```python
from build123d import *

# Parameters (mm, degrees)
F0_R     = 9.3155
F1_DEPTH = 11
F2_R     = 10.4775
F3_DEPTH = 19
F4_R     = 9.3155
F5_DEPTH = 11


with BuildPart() as f1:
    # F0 (on Front) → F1 (new body)
    with BuildSketch(Plane.XZ):
        Polygon((13.5, -5.591883), (13.5, 5.591883), (5.591883, 13.5), (-5.591883, 13.5), (-13.5, 5.591883), (-13.5, -5.591883), (-5.591883, -13.5), (5.591883, -13.5), align=None)
        Circle(F0_R, mode=Mode.SUBTRACT)
    extrude(amount=F1_DEPTH)

    # F2 (on face) → F3 (join)
    with BuildSketch(Plane(origin=(0, 0, 0), x_dir=(-1, 0, 0), z_dir=(0, 1, 0))):
        Polygon((21, -8.698485), (21, 8.698485), (8.698485, 21), (-8.698485, 21), (-21, 8.698485), (-21, -8.698485), (-8.698485, -21), (8.698485, -21), align=None)
        Circle(F2_R, mode=Mode.SUBTRACT)
    extrude(amount=F3_DEPTH)

    # F4 (on face) → F5 (join)
    with BuildSketch(Plane(origin=(0, 19, 0), x_dir=(-1, 0, 0), z_dir=(0, 1, 0))):
        Polygon((13.5, -5.591883), (13.5, 5.591883), (5.591883, 13.5), (-5.591883, 13.5), (-13.5, 5.591883), (-13.5, -5.591883), (-5.591883, -13.5), (5.591883, -13.5), align=None)
        Circle(F4_R, mode=Mode.SUBTRACT)
    extrude(amount=F5_DEPTH)


solid = f1.part
```
Work out the finished part from the listing and answer in its coordinate system (mm). A direction names the side the tool comes from. Give positions to 0.01 mm unless a question says otherwise; leave off trailing zeros. Order: outer loops, then holes, each group sorted by start corner. A loop starts at its lowest first (then second) coordinate and runs counter-clockwise, first axis right, second up. Notation, with made-up numbers: (66.5, -9.5) - (100.5, -9.5) arc R11 cw to (100.5, -3.5) - close; hole circle Ø8 at (24.25, 49). An arc over 180 degrees is marked (long way). One line per item, written item: value. Start each with the question number.
1. Section A-A, the plane x = 0 is taken. Write down the section's boundary in (y, z).
2. Section C-C, the plane y = -4 is taken. Write down the section's boundary in (x, z), then the cut area to 3 significant figures.
3. Consider line 1 (Z direction, x = 0, y = -5.5); line 2 (Z direction, x = 0, y = 10.5); line 3 (X direction, y = 24.5, z = 1). Determine where each line is inside the solid, lowest interval first.
4. Each of these flat-tipped pins is pushed along its axis until it touches: pin 1 Ø10 at (y, z) = (25, 8) entering from -X; pin 2 Ø3 at (x, y) = (0, -6) entering from -Z; pin 3 Ø3 at (x, y) = (13.5, 11) entering from +Z; pin 4 Ø6.5 at (x, z) = (0, 3) entering from +Y. Where does it stop, or does it pass through?
5. Which of the six approach directions +Z, -Z, +X, -X, +Y, -Y give full straight-line access (tool end or side, diameter ignored) to faces 4 (the face through (9.49, 24.42, 9.6)), 5 (the face through (-9.49, -5.42, 9.6)), 6 (the face through (0, -5, -13.5))?
6. Section B-B, the plane z = 0 is taken. Write down the section's boundary in (x, y), then the cut area to 3 significant figures.
7. Section D-D, the plane y = 17 is taken. Write down the section's boundary in (x, z) (1 decimal), then the cut area to 3 significant figures.
8. For a pull along Y with two mould halves and no side action, classify faces 1 (the face through (9.6, 24.42, -9.49)), 2 (the face through (9, 19, -4)), 3 (the face through (10, 0, 10)) as released by +Y, released by -Y, zero draft, split by the parting line, or undercut.
Filled sheet:
1. outline: (-11, -13.5) - (0, -13.5) - (0, -21) - (19, -21) - (19, -13.5) - (30, -13.5) - (30, -9.32) - (19, -9.32) - (19, -10.48) - (0, -10.48) - (0, -9.32) - (-11, -9.32) - close; (-11, 9.32) - (0, 9.32) - (0, 10.48) - (19, 10.48) - (19, 9.32) - (30, 9.32) - (30, 13.5) - (19, 13.5) - (19, 21) - (0, 21) - (0, 13.5) - (-11, 13.5) - close
2. outline: (-13.5, -5.59) - (-5.59, -13.5) - (5.59, -13.5) - (13.5, -5.59) - (13.5, 5.59) - (5.59, 13.5) - (-5.59, 13.5) - (-13.5, 5.59) - close; hole circle Ø18.63 at (0, 0)
2. area: 331 mm²
3. line 1: -13.5 to -9.32, 9.32 to 13.5
3. line 2: -21 to -10.48, 10.48 to 21
3. line 3: -13.5 to -9.26, 9.26 to 13.5
4. pin 1: x = -13.5
4. pin 2: z = -13.5
4. pin 3: z = 17.7
4. pin 4: through
5. face 4: +Z, +X, +Y
5. face 5: +Z, -X, -Y
5. face 6: -Z, +X, -X, -Y
6. outline: (-21, 0) - (-13.5, 0) - (-13.5, -11) - (-9.32, -11) - (-9.32, 0) - (-10.48, 0) - (-10.48, 19) - (-9.32, 19) - (-9.32, 30) - (-13.5, 30) - (-13.5, 19) - (-21, 19) - close; (9.32, -11) - (13.5, -11) - (13.5, 0) - (21, 0) - (21, 19) - (13.5, 19) - (13.5, 30) - (9.32, 30) - (9.32, 19) - (10.48, 19) - (10.48, 0) - (9.32, 0) - close
6. area: 584 mm²
7. outline: (-21, -8.7) - (-8.7, -21) - (8.7, -21) - (21, -8.7) - (21, 8.7) - (8.7, 21) - (-8.7, 21) - (-21, 8.7) - close; hole circle Ø21 at (0, 0)
7. area: 1,120 mm²
8. face 1: zero draft
8. face 2: undercut
8. face 3: released by -Y
